```python
from build123d import *


with BuildPart() as f1:
    # F0 (on Front) → F1 (revolve)
    with BuildSketch(Plane.XZ):
        with BuildLine():
            Line((0, 61), (0, 0))
            Line((0, 0), (35, 0))
            Line((35, 0), (35, 10))
            Line((35, 10), (20, 10))
            Line((20, 10), (20, 40))
            Line((20, 40), (50, 40))
            Line((50, 40), (50, 70))
            ThreePointArc((50, 70), (49.267767, 71.767767), (47.5, 72.5))
            Line((47.5, 72.5), (45, 72.5))
            Line((45, 72.5), (45, 61))
            Line((45, 61), (0, 61))
        make_face()
        with BuildLine():
            Line((-35, 0), (0, 0))
            Line((0, 0), (0, 61))
            Line((0, 61), (-45, 61))
            Line((-45, 61), (-45, 72.5))
            Line((-45, 72.5), (-47.5, 72.5))
            ThreePointArc((-47.5, 72.5), (-49.267767, 71.767767), (-50, 70))
            Line((-50, 70), (-50, 40))
            Line((-50, 40), (-20, 40))
            Line((-20, 40), (-20, 10))
            Line((-20, 10), (-35, 10))
            Line((-35, 10), (-35, 0))
        make_face()
    revolve(axis=Axis((25.468834, 0, -717.5), (1, 0, 0)))


solid = f1.part
```
The listing builds one solid part. Answer for the finished solid, in the listing's coordinates (mm). A direction names the side the tool comes from. Round coordinates to 2 decimals unless told otherwise and drop trailing zeros.
1) For a pull along X with two mould halves and no side action, classify faces 1 (the face through (45, 523, -136)), 2 (the face through (50, -645, -305)), 3 (the face through (-46.27, -533.92, -1299.76)) as released by +X, released by -X, zero draft, split by the parting line, or undercut.
Outcome:
face 1: undercut
face 2: released by +X
face 3: zero draft
2) For faces 4 (the face through (-45, 523, -1299)), 5 (the face through (-35, 482, -182)), 6 (the face through (20, -284, -41)), determine the directions among +Z, -Z, +X, -X, +Y, -Y from which every point of the face is accessible in a straight line to the end or side of a thin tool.
Outcome:
face 4: none
face 5: -X
face 6: +X
3) Consider line 1 (Y direction, x = -33, z = -717.5); line 2 (Z direction, x = 26, y = 0); line 3 (Y direction, x = 16, z = -717.5). Determine where each line is inside the solid, lowest interval first.
Outcome:
line 1: y = -778.5 to -757.5, -727.5 to -717.5, 717.5 to 727.5, 757.5 to 778.5
line 2: z = -1496 to -1475, -1445 to -1435, 0 to 10, 40 to 61
line 3: y = -778.5 to -717.5, 717.5 to 778.5
4) Given P1, Ø12, axis at x = 0.5, y = 498, coming from the -Z side; P2, Ø4, axis at x = -1, y = -76.5, coming from the -Z side; P3, Ø3, axis at x = -28.5, y = -409.5, coming from the -Z side, each flat-ended and moving along its own axis, determine where each tip first touches the part or whether it passes through.
Outcome:
P1: stops at z = -1320.82
P2: stops at z = -1492.43
P3: stops at z = -1380.52
